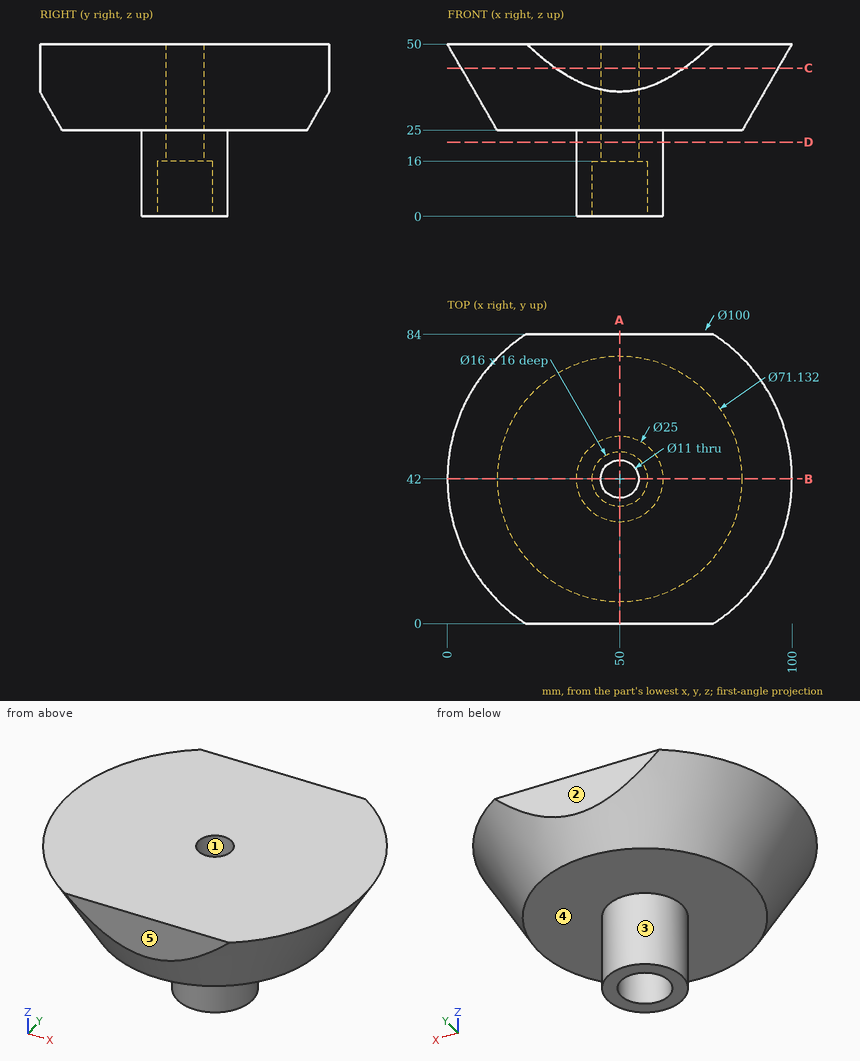
Part print with two shaded views. Sizes in mm from the minimum x, y, z corner. A direction names the side the tool comes from. Give positions to 0.01 mm unless a question says otherwise; leave off trailing zeros. Order: outer loops, then holes, each group sorted by start corner. A loop starts at its lowest first (then second) coordinate and runs counter-clockwise, first axis right, second up.
1) Saw through at C-C, the plane z = 43. Write the cut outline in (x, y).
2) Saw through at A-A, the plane x = 50. Write the cut outline in (y, z).
3) Wall check: probe 1 along Y at (x, z) = (50, 10.25); probe 2 along Z at (x, y) = (21, 46); probe 3 along Y at (x, z) = (46.5, 11) (1 decimal). Give the ranges that are in metal, low to high.
4) Mould opens along Y. For the marked faces 1, 2 and 3 say: +Y half, -Y half, draft (parallel to the pull), parting line (faces both ways), or undercut.
5) Saw through at D-D, the plane z = 21.5. Write the cut outline in (x, y), then the cut area to 3 significant figures.
6) Saw through at B-B, the plane y = 42. Write the cut outline in (x, z).
7) Pin check, flat tips, straight feed: pin 1 (8 mm diameter, centred on y = 32.5, z = 5.5, fed in from +X) (1 decimal); pin 2 (5 mm diameter, centred on x = 46.5, y = 41.5, fed in from -Z); pin 3 (5 mm diameter, centred on x = 72, y = 56, fed in from -Z); pin 4 (10 mm diameter, centred on y = 62, z = 6.5, fed in from -X). Stop position of each tip, or through.
8) 3-axis set-ups, long thin cutter, end or side, ignore diameter. For the marked faces 4 and 5: which of +Z, -Z, +X, -X, +Y, -Y reach the whole face in a straight line?
Computed:
1. outline: (31.34, 0) - (68.66, 0) arc R45.96 ccw to (68.66, 84) - (31.34, 84) arc R45.96 ccw to start; hole circle Ø11 at (50, 42)
2. outline: (0, 36.14) - (6.43, 25) - (29.5, 25) - (29.5, 0) - (34, 0) - (34, 16) - (36.5, 16) - (36.5, 50) - (0, 50) - close; (47.5, 16) - (50, 16) - (50, 0) - (54.5, 0) - (54.5, 25) - (77.57, 25) - (84, 36.14) - (84, 50) - (47.5, 50) - close
3. probe 1: y = 29.5 to 34, 50 to 54.5
3. probe 2: z = 25 to 50
3. probe 3: y = 30 to 34.8, 49.2 to 54
4. face 1: undercut
4. face 2: +Y half
4. face 3: parting line
5. outline: circle Ø25 at (50, 42); hole circle Ø11 at (50, 42)
5. area: 396 mm2
6. outline: (0, 50) - (14.43, 25) - (37.5, 25) - (37.5, 0) - (42, 0) - (42, 16) - (44.5, 16) - (44.5, 50) - close; (55.5, 16) - (58, 16) - (58, 0) - (62.5, 0) - (62.5, 25) - (85.57, 25) - (100, 50) - (55.5, 50) - close
7. pin 1: stops at x = 61.2
7. pin 2: stops at z = 16
7. pin 3: stops at z = 25
7. pin 4: passes through
8. face 4: -Z
8. face 5: +Z, -Z, +X, -X, -Y
